Here's how the part is built. I have some questions about the finished solid (model axes, mm). A direction names the side the tool comes from. Round coordinates to 2 decimals unless told otherwise and drop trailing zeros. Write each loop counter-clockwise with the first axis right and the second up, starting at its lowest first coordinate (ties: lowest second). Pieces come first, ordered by that corner, then holes. Notation, with made-up numbers: (10, 75.5) - (58, 75.5) arc R13 cw to (58, 82.5) - close; hole circle Ø5 at (-11, 48). An arc over 180 degrees is marked (long way). Use one line per item in the form item = value. Start each with the question number.
1. I want a section at A-A, the plane y = 12.5. List the corners of the cut face in (x, z) for me, plus the area to 3 significant figures.
2. Will these pins go through, and if not, where does the flat tip stop? pin 1 (0.8 mm diameter, centred on x = 25, y = 8.5, fed in from -Z); pin 2 (2 mm diameter, centred on y = 12, z = -5.5, fed in from -X); pin 3 (0.5 mm diameter, centred on y = 9, z = -2, fed in from -X).
3. I want a section at B-B, the plane x = 0. List the corners of the cut face in (y, z) for me.
4. If I drill on line 1 along Y through (x, z) = (0, 3.5); line 2 along Z through (x, y) = (-1, 2); line 3 along Y through (x, z) = (-24, 2), over which ranges is the centre line in solid material (lowest first)?
5. Which directions (+Z, -Z, +X, -X, +Y, -Y) give clear straight access to the entire face, cutting with the end or side of a thin tool? Please do faces 4 (the cylindrical face through (-22.35, 12.32, -2.78)), 5 (the flat face through (23, 9.8, 0)), 6 (the flat face through (0, 13, 1.969)), 7 (the flat face through (23, 8.3, 0)).
6. I want a section at D-D, the plane y = 9. State how many separate pieces and enclosed holes the cut face has, plus the area to 3 significant figures.
7. I want a section at C-C, the plane z = 0.25. List the corners of the cut face in (x, y) for me.
8. We'd pull the mould along Z, two halves only. Please class faces 1 (the flat face through (0, 1, 8.969)), 2 (the flat face through (0, 0, 0)), 3 (the flat face through (-22, 8.3, 0)): +Z half, -Z half, draft (parallel to the pull), parting line (faces both ways), or undercut.
```python
from build123d import *

# Parameters (mm, degrees)
SKETCH1_R           = 3
BOSS_EXTRUDE1_DEPTH = 25
SKETCH3_R           = 11
CUT_EXTRUDE1_DEPTH  = 7
BOSS_EXTRUDE2_START = -1.5
BOSS_EXTRUDE2_DEPTH = 1.5
BOSS_EXTRUDE3_START = -1.5
BOSS_EXTRUDE3_DEPTH = 1.5


with BuildPart() as part:
    # Sketch1 → Boss-Extrude1 (new body)
    with BuildSketch(Plane(origin=(0, 0, 0), x_dir=(1, 0, 0), z_dir=(0, 1, 0))):
        with BuildLine():
            Line((-22.480683045, -8.968703758), (22.619316955, -8.968703758))
            ThreePointArc((22.619316955, -8.968703758), (31.369316462, -0.218703512), (22.619316462, 8.531296242))
            Line((22.619316462, 8.531296242), (-22.480682552, 8.531296242))
            ThreePointArc((-22.480682552, 8.531296242), (-31.230682552, -0.218703512), (-22.480683045, -8.968703758))
        make_face()
        with Locations(Location((-22.480682552, -0.218703758, 0), (0, 0, 270))):
            Circle(SKETCH1_R, mode=Mode.SUBTRACT)
        with Locations(Location((22.619316462, -0.218703758, 0), (0, 0, 270))):
            Circle(SKETCH1_R, mode=Mode.SUBTRACT)
    extrude(amount=BOSS_EXTRUDE1_DEPTH)

    # Sketch3 → Cut-Extrude1 (cut)
    with BuildSketch(Plane.XY.offset(8.968703758)):
        with Locations((0, 12.5)):
            Circle(SKETCH3_R)
    extrude(amount=-CUT_EXTRUDE1_DEPTH, mode=Mode.SUBTRACT)

    # Sketch4 → Boss-Extrude2 (add)
    with BuildSketch(Plane(origin=(0, 9.8, 0), x_dir=(1, 0, 0), z_dir=(0, 1, 0)).offset(BOSS_EXTRUDE2_START)):
        with BuildLine():
            Line((-20.730682552, 2.217994828), (-20.730682552, 1.531296242))
            Line((-20.730682552, 1.531296242), (-20.043983966, 1.531296242))
            ThreePointArc((-20.043983966, 1.531296242), (-19.480682552, -0.218703758), (-20.043983966, -1.968703758))
            Line((-20.043983966, -1.968703758), (-20.730682552, -1.968703758))
            Line((-20.730682552, -1.968703758), (-20.730682552, -2.655402344))
            ThreePointArc((-20.730682552, -2.655402344), (-22.480682552, -3.218703758), (-24.230682552, -2.655402344))
            Line((-24.230682552, -2.655402344), (-24.230682552, -1.968703758))
            Line((-24.230682552, -1.968703758), (-24.917381138, -1.968703758))
            ThreePointArc((-24.917381138, -1.968703758), (-25.480682552, -0.218703758), (-24.917381138, 1.531296242))
            Line((-24.917381138, 1.531296242), (-24.230682552, 1.531296242))
            Line((-24.230682552, 1.531296242), (-24.230682552, 2.217994828))
            ThreePointArc((-24.230682552, 2.217994828), (-22.480682552, 2.781296242), (-20.730682552, 2.217994828))
        make_face()
    extrude(amount=BOSS_EXTRUDE2_DEPTH)

    # Sketch5 → Boss-Extrude3 (add)
    with BuildSketch(Plane(origin=(0, 9.8, 0), x_dir=(1, 0, 0), z_dir=(0, 1, 0)).offset(BOSS_EXTRUDE3_START)):
        with BuildLine():
            Line((24.369316462, 2.217994828), (24.369316462, 1.531296242))
            Line((24.369316462, 1.531296242), (25.056015049, 1.531296242))
            ThreePointArc((25.056015049, 1.531296242), (25.619316462, -0.218703758), (25.056015049, -1.968703758))
            Line((25.056015049, -1.968703758), (24.369316462, -1.968703758))
            Line((24.369316462, -1.968703758), (24.369316462, -2.655402344))
            ThreePointArc((24.369316462, -2.655402344), (22.619316462, -3.218703758), (20.869316462, -2.655402344))
            Line((20.869316462, -2.655402344), (20.869316462, -1.968703758))
            Line((20.869316462, -1.968703758), (20.182617876, -1.968703758))
            ThreePointArc((20.182617876, -1.968703758), (19.619316462, -0.218703758), (20.182617876, 1.531296242))
            Line((20.182617876, 1.531296242), (20.869316462, 1.531296242))
            Line((20.869316462, 1.531296242), (20.869316462, 2.217994828))
            ThreePointArc((20.869316462, 2.217994828), (22.619316462, 2.781296242), (24.369316462, 2.217994828))
        make_face()
    extrude(amount=BOSS_EXTRUDE3_DEPTH)


solid = part.part
```
Model answer:
q1.outline = (-22.48, -8.53) - (22.62, -8.53) arc R8.75 ccw to (22.62, 8.97) - (11, 8.97) - (11, 1.97) - (-11, 1.97) - (-11, 8.97) - (-22.48, 8.97) arc R8.75 ccw to start; hole circle Ø6 at (-22.48, 0.22); hole circle Ø6 at (22.62, 0.22)
q1.area = 819 mm2
q2.pin_1 = -8.3
q2.pin_2 = -29.85
q2.pin_3 = -31.01
q3.outline = (0, -8.53) - (25, -8.53) - (25, 8.97) - (23.5, 8.97) - (23.5, 1.97) - (1.5, 1.97) - (1.5, 8.97) - (0, 8.97) - close
q4.line_1 = 0 to 1.5, 23.5 to 25
q4.line_2 = -8.53 to 1.97
q4.line_3 = 8.3 to 9.8
q5.face_4 = none
q5.face_5 = +Y
q5.face_6 = +Z
q5.face_7 = -Y
q6.separate_pieces = 1
q6.enclosed_holes = 8
q6.area = 882 mm2
q7.outline = (-31.23, 0) - (-25.48, 0) - (-25.48, 8.3) - (-19.48, 8.3) - (-19.48, 0) - (19.62, 0) - (19.62, 8.3) - (25.62, 8.3) - (25.62, 0) - (31.37, 0) - (31.37, 25) - (25.62, 25) - (25.62, 9.8) - (19.62, 9.8) - (19.62, 25) - (-19.48, 25) - (-19.48, 9.8) - (-25.48, 9.8) - (-25.48, 25) - (-31.23, 25) - close
q8.face_1 = +Z half
q8.face_2 = draft
q8.face_3 = undercut
